```python
from build123d import *

# Parameters (mm, degrees)
SKETCH1_R           = 24
BOSS_EXTRUDE1_DEPTH = 4
SKETCH4_R           = 2
CUT_EXTRUDE3_DEPTH  = 442.841600576
SKETCH7_R           = 24
SKETCH7_R_2         = 21
BOSS_EXTRUDE3_DEPTH = 4
SKETCH8_R           = 2
CUT_EXTRUDE5_DEPTH  = 442.841600576


with BuildPart() as part:
    # Sketch1 → Boss-Extrude1 (new body)
    with BuildSketch(Plane(origin=(0, 0, 0), x_dir=(0, 0, -1), z_dir=(1, 0, 0))):
        with BuildLine():
            Line((0, 58), (380, 58))
            ThreePointArc((380, 58), (438, 0), (380, -58))
            Line((380, -58), (0, -58))
            ThreePointArc((0, -58), (-58, 0), (0, 58))
        make_face()
        Circle(SKETCH1_R, mode=Mode.SUBTRACT)
        with Locations((380, 0)):
            Circle(SKETCH1_R, mode=Mode.SUBTRACT)
    extrude(amount=BOSS_EXTRUDE1_DEPTH)

    # Sketch4 → Cut-Extrude3 (cut, through all)
    with BuildSketch(Plane.ZY):
        with Locations((0, 32.5)):
            Circle(SKETCH4_R)
        with Locations((32.5, 0)):
            Circle(SKETCH4_R)
        with Locations((0, -32.5)):
            Circle(SKETCH4_R)
        with Locations((-32.5, 0)):
            Circle(SKETCH4_R)
    extrude(amount=-CUT_EXTRUDE3_DEPTH, mode=Mode.SUBTRACT)

    # Sketch7 → Boss-Extrude3 (add)
    with BuildSketch(Plane.ZY):
        with Locations((-380, 0)):
            Circle(SKETCH7_R)
        with Locations((-380, 0)):
            Circle(SKETCH7_R_2, mode=Mode.SUBTRACT)
    extrude(amount=-BOSS_EXTRUDE3_DEPTH)

    # Sketch8 → Cut-Extrude5 (cut, through all)
    with BuildSketch(Plane.ZY):
        with Locations((-380, 26)):
            Circle(SKETCH8_R)
        with Locations((-354, 0)):
            Circle(SKETCH8_R)
        with Locations((-380, -26)):
            Circle(SKETCH8_R)
        with Locations((-406, 0)):
            Circle(SKETCH8_R)
    extrude(amount=-CUT_EXTRUDE5_DEPTH, mode=Mode.SUBTRACT)


solid = part.part
```
Here's how the part is built. I have some questions about the finished solid (model axes, mm). Give positions to 0.01 mm unless a question says otherwise; leave off trailing zeros. Order: outer loops, then holes, each group sorted by start corner. A loop starts at its lowest first (then second) coordinate and runs counter-clockwise, first axis right, second up. Notation, with made-up numbers: M 4.25,86 L 47.25,86 A31 cw 47.25,121 Z; hole C 49.5,28 d11. An arc over 180 degrees is marked long. Use a Markdown table: item, result. Add a question column.
1. Suppose I cut it at A-A (x = 0.85). Give the number of separate pieces and of enclosed holes in the cut face, and give its area (3 significant figures).
2. I need wall thicknesses on probe 1 along Y at (x, z) = (2, -380); probe 2 along Y at (x, z) = (2.75, 0); probe 3 along Z at (x, y) = (2.1, -17). Which ranges of each line are inside material? Lowest first, please. Write a range as from..to.
3. Suppose I cut it at B-B (y = -10). List the corners of the cut face in (x, z) for me, and give its area (3 significant figures).
4. For pin 1 Ø1 at (x, y) = (1.5, -14.5) entering from -Z (3 decimals), with a flat end and sliding along its axis, tell me the tip position at first contact or that it passes through.
5. Suppose I cut it at D-D (y = 41). List the corners of the cut face in (x, z) for me.
6. Suppose I cut it at C-C (z = -391.5). List the corners of the cut face in (x, y) for me.
7. If we mould it in two halves opening along Y, with no side actions, what happens to faces 1 (the cylindrical face through (1.972, 1.275, -437.986)), 2 (the cylindrical face through (1.97, 6.31, -359.97)), 3 (the flat face through (4, 1, -193))? For each: +Y half, -Y half, draft (parallel to the pull), parting line (faces both ways), or undercut.
Results list:
| question | item | result |
|---|---|---|
| 1 | separate pieces | 1 |
| 1 | enclosed holes | 10 |
| 1 | area | 51,400 mm² |
| 2 | probe 1 | y = -58..-28, -24..-21, 21..24, 28..58 |
| 2 | probe 2 | y = -58..-34.5, -30.5..-24, 24..30.5, 34.5..58 |
| 2 | probe 3 | z = -435.45..-392.33, -367.67..-16.94, 16.94..55.45 |
| 3 | outline | M 0,-437.13 L 4,-437.13 L 4,-398.47 L 0,-398.47 Z; M 0,-361.53 L 4,-361.53 L 4,-21.82 L 0,-21.82 Z; M 0,21.82 L 4,21.82 L 4,57.13 L 0,57.13 Z |
| 3 | area | 1,650 mm² |
| 4 | pin 1 | stops at z = -436.285 |
| 5 | outline | M 0,-421.02 L 4,-421.02 L 4,41.02 L 0,41.02 Z |
| 6 | outline | M 0,-56.85 L 4,-56.85 L 4,-17.57 L 0,-17.57 Z; M 0,17.57 L 4,17.57 L 4,56.85 L 0,56.85 Z |
| 7 | face 1 | parting line |
| 7 | face 2 | undercut |
| 7 | face 3 | draft |
